Build history of the part. All positions in model axes, mm. A direction names the side the tool comes from. Round coordinates to 2 decimals unless told otherwise and drop trailing zeros. Write each loop counter-clockwise with the first axis right and the second up, starting at its lowest first coordinate (ties: lowest second). Pieces come first, ordered by that corner, then holes.
Item 1: Drop flat-ended pins along their axis: pin 1 Ø8 at (x, y) = (-79.5, -10) entering from -Z; pin 2 Ø2 at (y, z) = (-5.5, 60.5) entering from -X; pin 3 Ø8 at (x, y) = (96.5, -3.5) entering from -Z; pin 4 Ø5 at (x, z) = (-85, 13.5) entering from +Y. Give the stop position or say it passes through.
Item 2: Band-saw the part on D-D, the plane z = 28. Write the cut outline in (x, y).
Item 3: 3-axis set-ups, long thin cutter, end or side, ignore diameter. For faces 1 (the flat face through (-83, -4.054, 13)), 2 (the flat face through (-83, -14.054, 13)), 3 (the flat face through (-83, -9, 8)), 4 (the flat face through (121.2, -9, 60)): which of +Z, -Z, +X, -X, +Y, -Y reach the whole face in a straight line?
Item 4: Band-saw the part on C-C, the plane x = 92.5. Write the cut outline in (y, z).
Item 5: Band-saw the part on B-B, the plane y = -10.25. Write the cut outline in (x, z).
Item 6: Band-saw the part on A-A, the plane z = 16. Write the cut outline in (x, y), then the cut area to 3 significant figures.
Item 7: Wall check: probe 1 along X at (y, z) = (-17.5, 75); probe 2 along X at (y, z) = (-1.75, 5); probe 3 along Z at (x, y) = (-32, -4.25). Give the ranges that are in metal, low to high.
```python
from build123d import *

# Parameters (mm, degrees)
F0_W     = 190
F0_H     = 19.5
F0_W_2   = 10
F1_DEPTH = 25
F2_W     = 10
F2_H     = 19.5
F3_DEPTH = 70
F4_W     = 10
F4_H     = 10
F5_DEPTH = 28


with BuildPart() as f1:
    # F0 (on Top) → F1 (new body)
    with BuildSketch(Plane.XY):
        with Locations((26.199683, -9.304239)):
            Rectangle(F0_W, F0_H)
        with Locations((126.199683, -9.304239)):
            Rectangle(F0_W_2, F0_H)
    extrude(amount=F1_DEPTH)

    # F2 (on face) → F3 (join)
    with BuildSketch(Plane.XY.offset(25)):
        with Locations((126.199683, -9.304239)):
            Rectangle(F2_W, F2_H)
    extrude(amount=F3_DEPTH)

    # F4 (on face) → F5 (join)
    with BuildSketch(Plane(origin=(-68.800317, 0, 0), x_dir=(0, -1, 0), z_dir=(-1, 0, 0))):
        with Locations((9.054239, 13)):
            Rectangle(F4_W, F4_H)
    extrude(amount=F5_DEPTH)


solid = f1.part
```
Results:
1. pin 1: stops at z = 8
1. pin 2: stops at x = 121.2
1. pin 3: stops at z = 0
1. pin 4: stops at y = -4.05
2. outline: (121.2, -19.05) - (131.2, -19.05) - (131.2, 0.45) - (121.2, 0.45) - close
3. face 1: +Z, -Z, -X, +Y
3. face 2: +Z, -Z, -X, -Y
3. face 3: -Z, -X, +Y, -Y
3. face 4: +Z, -X, +Y, -Y
4. outline: (-19.05, 0) - (0.45, 0) - (0.45, 25) - (-19.05, 25) - close
5. outline: (-96.8, 8) - (-68.8, 8) - (-68.8, 0) - (131.2, 0) - (131.2, 95) - (121.2, 95) - (121.2, 25) - (-68.8, 25) - (-68.8, 18) - (-96.8, 18) - close
6. outline: (-96.8, -14.05) - (-68.8, -14.05) - (-68.8, -19.05) - (131.2, -19.05) - (131.2, 0.45) - (-68.8, 0.45) - (-68.8, -4.05) - (-96.8, -4.05) - close
6. area: 4,180 mm2
7. probe 1: x = 121.2 to 131.2
7. probe 2: x = -68.8 to 131.2
7. probe 3: z = 0 to 25
